Geometry check sheet. Reference: the model listing, model coordinates, mm. A direction names the side the tool comes from. Give positions to 0.01 mm unless a question says otherwise; leave off trailing zeros. Loops run counter-clockwise (first coordinate to the right, second up) from the corner with the lowest first, then second, coordinate; pieces in that order, holes last. Notation, with made-up numbers: (-32, 79.25) -> (-23, 79.25) arc R25 ccw to (-23, 117.25) -> close; hole circle Ø11 at (-35, -22.75). An arc over 180 degrees is marked (long way). Answer as a JSON object with one key per item and string values.
from build123d import *

# Parameters (mm, degrees)
BOSS_EXTRUDE1_DEPTH = 20
FILLET1_R           = 10
CUT_EXTRUDE1_REACH  = 102
SKETCH5_R           = 28


with BuildPart() as part:
    # Sketch1 → Revolve1 (revolve)
    with BuildSketch(Plane.XY):
        Polygon((0, 0), (40, 0), (40, 34), (35, 34), (35, 46), (40, 46), (40, 80), (0, 80), align=None)
    revolve(axis=Axis((0, 103.412132622, 0), (0, -1, 0)))

    # Sketch2 → Boss-Extrude1 (add)
    with BuildSketch(Plane(origin=(0, 80, 0), x_dir=(1, 0, 0), z_dir=(0, 1, 0))):
        Polygon((-28.321671813, 50), (28.321671813, 50), (54.938741093, 0), (28.321671813, -50), (-28.321671813, -50), (-54.938741093, 0), align=None)
    extrude(amount=BOSS_EXTRUDE1_DEPTH)

    # Fillet1
    fillet1_edges = [part.edges().sort_by_distance(p)[0] for p in [
        (-41.630206453, 100, -25),
        (-41.630206453, 100, 25),
        (0, 100, 50),
        (41.630206453, 100, 25),
        (41.630206453, 100, -25),
        (0, 100, -50),
    ]]
    fillet(fillet1_edges, radius=FILLET1_R)

    # Sketch5 → Cut-Extrude1 (cut, up to next)
    with BuildSketch(Plane.XZ, mode=Mode.PRIVATE) as cut_extrude1_sk1:
        Circle(SKETCH5_R)
    cut_extrude1_tool1 = extrude(cut_extrude1_sk1.sketch, amount=-CUT_EXTRUDE1_REACH, mode=Mode.PRIVATE) & part.part
    add(cut_extrude1_tool1.solids().sort_by_distance((0, 0, 0))[0], mode=Mode.SUBTRACT)


solid = part.part
1) Tool access check on faces 4 (the face through (0.2, 46, -35.4)), 5 (the face through (-39.16, 97.15, 23.24)), 6 (the face through (-8.67, 63.24, -39.05)). Record the directions out of +Z, -Z, +X, -X, +Y, -Y that give a thin tool (end or side, any length) a straight path to the whole face; none if there is none.
Geometry check:
{"face 4": "none", "face 5": "+Z, -X, +Y", "face 6": "-Y"}
2) Section check B-B on y = 71.5. Record the cut outline in (x, z), plus the area to 3 significant figures.
Geometry check:
{"outline": "circle Ø80 at (0, 0); hole circle Ø56 at (0, 0)", "area": "2,560 mm2"}
3) Section check C-C on x = -16. Record the cut outline in (y, z), plus the area to 3 significant figures.
Geometry check:
{"outline": "(0, -36.66) -> (34, -36.66) -> (34, -31.13) -> (46, -31.13) -> (46, -36.66) -> (80, -36.66) -> (80, -50) -> (90, -50) arc R10 ccw to (100, -40) -> (100, -22.98) -> (0, -22.98) -> close; (0, 22.98) -> (100, 22.98) -> (100, 40) arc R10 ccw to (90, 50) -> (80, 50) -> (80, 36.66) -> (46, 36.66) -> (46, 31.13) -> (34, 31.13) -> (34, 36.66) -> (0, 36.66) -> close", "area": "3,090 mm2"}
4) Section check A-A on x = 0. Record the cut outline in (y, z), plus the area to 3 significant figures.
Geometry check:
{"outline": "(0, -40) -> (34, -40) -> (34, -35) -> (46, -35) -> (46, -40) -> (80, -40) -> (80, -50) -> (90, -50) arc R10 ccw to (100, -40) -> (100, -28) -> (0, -28) -> close; (0, 28) -> (100, 28) -> (100, 40) arc R10 ccw to (90, 50) -> (80, 50) -> (80, 40) -> (46, 40) -> (46, 35) -> (34, 35) -> (34, 40) -> (0, 40) -> close", "area": "2,640 mm2"}
5) Material ranges on line 1 along Z through (x, y) = (0, 74); line 2 along Y through (x, z) = (-16.5, 34); line 3 along Z through (x, y) = (0, 45), recorded low to high. Write a range as from..to.
Geometry check:
{"line 1": "z = -40..-28, 28..40", "line 2": "y = 0..34, 46..100", "line 3": "z = -35..-28, 28..35"}
6) Draft check along Y on faces 1 (the face through (-28, 40, -21)), 2 (the face through (-41.817, 84.93, -24.65)), 3 (the face through (-28.5, 100, -0.6)). Enter one of: pulls with the +Y half, pulls with the -Y half, needs draft (parallel to the pull), parting line crosses it, or undercut.
Geometry check:
{"face 1": "undercut", "face 2": "needs draft", "face 3": "pulls with the +Y half"}
7) Section check D-D on y = 93. Record the cut outline in (x, z).
Geometry check:
{"outline": "(-54.42, 0) -> (-28.05, -49.54) -> (28.05, -49.54) -> (54.42, 0) -> (28.05, 49.54) -> (-28.05, 49.54) -> close; hole circle Ø56 at (0, 0)"}
8) Depth check by flat-ended pin: P1, Ø5, axis at y = 15, z = -5, coming from the -X side; P2, Ø1, axis at x = 12.5, y = 36, coming from the +Z side; P3, Ø5, axis at x = 43.5, z = -30.5, coming from the +Y side; P4, Ø4, axis at y = 76, z = -9, coming from the -X side. Enter the tip coordinate at first touch or a pass-through.
Geometry check:
{"P1": "stops at x = -39.92", "P2": "stops at z = 32.88", "P3": "passes through", "P4": "stops at x = -39.38"}
